from build123d import *

# Parameters (mm, degrees)
F1_DEPTH = 30
F3_DEPTH = 22.001
F4_DEPTH = 30


with BuildPart() as f1:
    # F0 (on Front) → F1 (new body)
    with BuildSketch(Plane.XZ):
        Polygon((0, 22), (0, 0), (50, 0), (50, 4), (12, 22), align=None)
    extrude(amount=-F1_DEPTH)

    # F2 (on face) → F3 (cut, through all)
    with BuildSketch(Plane(origin=(0, 0, 0), x_dir=(1, 0, 0), z_dir=(0, 0, -1))):
        Polygon((20, 0), (50, -16), (50, 0), align=None)
    extrude(amount=-F3_DEPTH, mode=Mode.SUBTRACT)

    # F2 (on face) → F4 (join)
    with BuildSketch(Plane(origin=(0, 0, 0), x_dir=(1, 0, 0), z_dir=(0, 0, -1))):
        Polygon((0, -30), (25, -30), (25, -25), (0, -10), align=None)
    extrude(amount=-F4_DEPTH)


solid = f1.part
Here's how the part is built. I have some questions about the finished solid (model axes, mm). A direction names the side the tool comes from. Coordinates: 2 decimals unless noted, no trailing zeros. Loops run counter-clockwise (first coordinate to the right, second up) from the corner with the lowest first, then second, coordinate; pieces in that order, holes last.
1. Imagine slicing it at B-B, the plane z = 2.75. Please give me the cut outline in (x, y), and give its area (3 significant figures).
2. For faces 1 (the flat face through (0, 15, 15)), 2 (the flat face through (25, 28, 23)), 3 (the flat face through (6, 7, 22)), which set-ups out of +Z, -Z, +X, -X, +Y, -Y let a thin tool reach every point of the face, with its end or its side?
3. For P1, Ø12, axis at y = 7.5, z = 18, coming from the -X side; P2, Ø2.5, axis at y = 28, z = 23, coming from the +X side; P3, Ø1.5, axis at x = 22.5, z = 3.5, coming from the -Y side; P4, Ø10, axis at y = 3.5, z = 18, coming from the +X side, each with a flat end and sliding along its axis, tell me the tip position at first contact or that it passes through.
4. Imagine slicing it at D-D, the plane z = 26.75. Please give me the cut outline in (x, y).
5. Imagine slicing it at C-C, the plane y = 23.5. Please give me the cut outline in (x, z).
6. I need wall thicknesses on L1, parallel to Y at x = 12, z = 25; L2, parallel to Y at x = 27.5, z = 13.25; L3, parallel to Z at x = 6.5, y = 8.5. Which ranges of each line are inside material? Lowest first, please.
7. Imagine slicing it at A-A, the plane x = 9.5. Please give me the cut outline in (y, z), and give its area (3 significant figures).
Taken from the geometry:
1. outline: (0, 0) - (20, 0) - (50, 16) - (50, 30) - (0, 30) - close
1. area: 1,260 mm2
2. face 1: +Z, -Z, -X, +Y, -Y
2. face 2: +Z, +X, +Y, -Y
2. face 3: +Z, +X, -Y
3. P1: stops at x = 0
3. P2: stops at x = 25
3. P3: stops at y = 0.93
3. P4: stops at x = 30.18
4. outline: (0, 10) - (25, 25) - (25, 30) - (0, 30) - close
5. outline: (0, 0) - (50, 0) - (50, 4) - (22.5, 17.03) - (22.5, 30) - (0, 30) - close
6. L1: y = 17.2 to 30
6. L2: y = 4 to 30
6. L3: z = 0 to 22
7. outline: (0, 0) - (30, 0) - (30, 30) - (15.7, 30) - (15.7, 22) - (0, 22) - close
7. area: 774 mm2
